The drawing under review shows one solid part. Ordinate dimensions are in mm from its lowest x, y, z. Coordinates: 2 decimals unless noted, no trailing zeros. Write each loop counter-clockwise with the first axis right and the second up, starting at its lowest first coordinate (ties: lowest second). Pieces come first, ordered by that corner, then holes.
1) Add section B-B, the plane z = 370. State the section outline as (x, y) points, then the cut area to 3 significant figures.
2) Add section A-A, the plane y = 6. State the section outline as (x, z) points, then the cut area to 3 significant figures.
3) For P1, Ø1, axis at x = 77.5, y = 10, coming from the -Z side; P2, Ø5, axis at y = 9.5, z = 277, coming from the +X side, all flat-tipped, find the tip position at first contact; note any pin that passes through.
4) For line 1 (X direction, y = 8, z = 270); line 2 (Z direction, x = 201.5, y = 7.25), list the stretches that pass through material, from the lowest coordinate up.
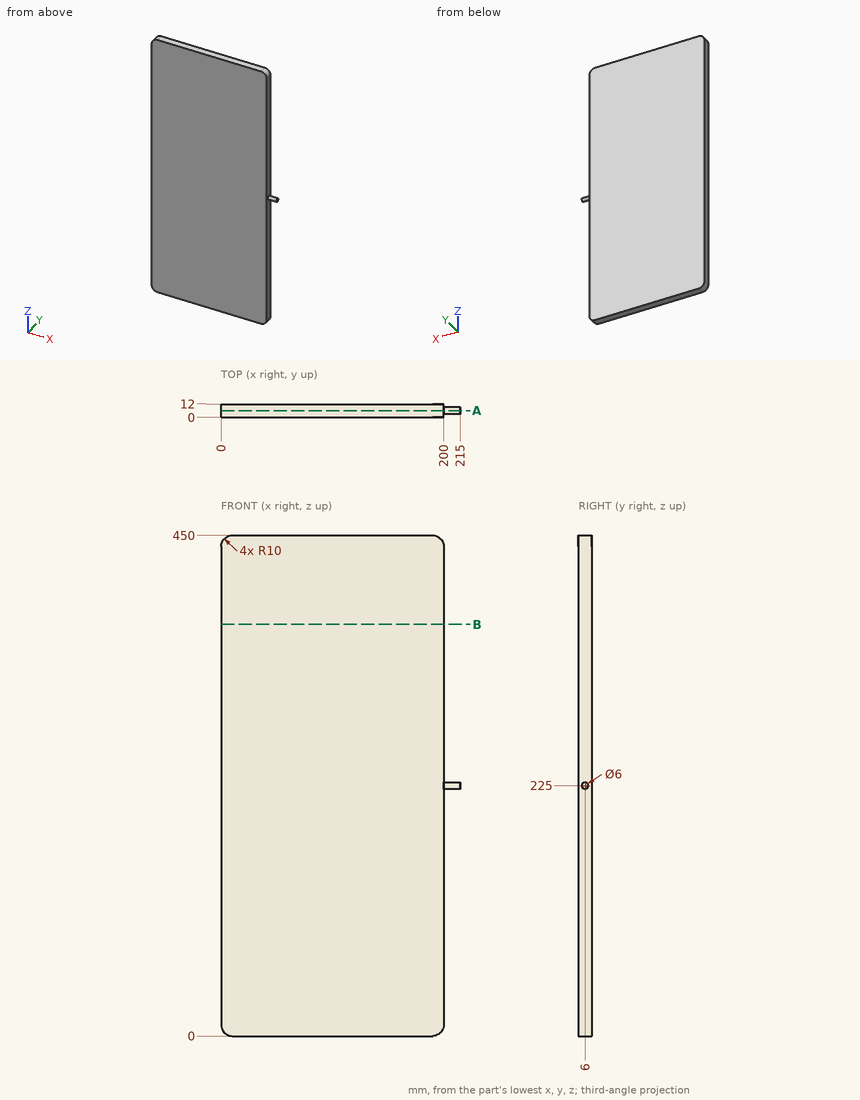
Geometry results:
1. outline: (0, 0) - (200, 0) - (200, 12) - (0, 12) - close
1. area: 2,400 mm2
2. outline: (0, 10) arc R10 ccw to (10, 0) - (190, 0) arc R10 ccw to (200, 10) - (200, 222) - (215, 222) - (215, 228) - (200, 228) - (200, 440) arc R10 ccw to (190, 450) - (10, 450) arc R10 ccw to (0, 440) - close
2. area: 90,000 mm2
3. P1: stops at z = 0
3. P2: stops at x = 200
4. line 1: x = 0 to 200
4. line 2: z = 222.27 to 227.73
